Check sheet for the modelled part. Datum: model origin and axes. Units: mm. Face numbers are marked on the shaded views. A direction names the side the tool comes from. Round coordinates to 2 decimals unless told otherwise and drop trailing zeros. Loops run counter-clockwise (first coordinate to the right, second up) from the corner with the lowest first, then second, coordinate; pieces in that order, holes last. Notation, with made-up numbers: (89, 18) - (138, 18) arc R9 ccw to (138, 32) - close; hole circle Ø10 at (-18.5, 52.25). An arc over 180 degrees is marked (long way). Answer in a Markdown table with one row per item. Add a question column.
(1) Mould release check, pull along X, two halves, no side actions. Record for the marked faces 4, 5 and 6: +X half, -X half, draft (parallel to the pull), parting line (faces both ways), or undercut.
(2) Cross-section at B-B on z = 1.35. Enter the section's corners in (x, y).
(3) Thickness scan on line 1 along Y through (x, z) = (-3, 2.1); line 2 along X through (y, z) = (-0.25, 3.3); line 3 along X through (y, z) = (1.75, 1.65). Record the ranges inside material, lowest first.
(4) Cross-section at C-C on y = 9. Enter the section's corners in (x, z), then the cut area to 3 significant figures.
(5) Access from +Z, -Z, +X, -X, +Y, -Y to the whole of each face (thin tool, end or side, straight path). Record for the marked faces 1, 2 and 3.
(6) Cross-section at A-A on x = -1.5. Enter the section's corners in (y, z).
(7) Cross-section at D-D on x = -11.25. Enter the section's corners in (y, z).
(8) Gauge pin test, flat ends, axial feed: pin 1 (9.5 mm diameter, centred on x = 0, y = 0, fed in from -Z); pin 2 (3 mm diameter, centred on x = -4, y = 10, fed in from -Z); pin 3 (1 mm diameter, centred on y = 7.5, z = 2, fed in from +X). Record the tip position at first contact, or that the pin passes through.
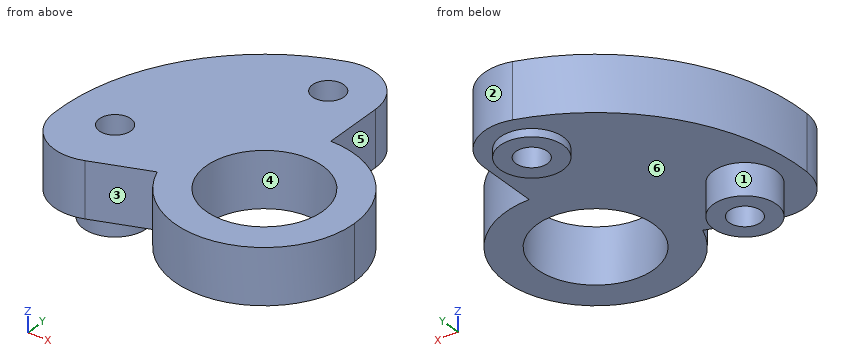
from build123d import *

# Parameters (mm, degrees)
SKETCH1_R           = 13
SKETCH1_R_2         = 5.7
SKETCH1_R_3         = 3.7
BOSS_EXTRUDE1_DEPTH = 3.5
CUT_EXTRUDE1_DEPTH  = 10
SKETCH3_R           = 1
CUT_EXTRUDE2_DEPTH  = 10
SKETCH5_R           = 1
CUT_EXTRUDE3_DEPTH  = 6
FILLET1_R           = 3
SKETCH6_R           = 2
SKETCH6_R_2         = 1
BOSS_EXTRUDE2_DEPTH = 2
SKETCH6_3_R         = 2
SKETCH6_3_R_2       = 1
BOSS_EXTRUDE3_DEPTH = 0.5


with BuildPart() as part:
    # Sketch1 → Boss-Extrude1 (new body)
    with BuildSketch(Plane.XY):
        Circle(SKETCH1_R)
        Circle(SKETCH1_R_2, mode=Mode.SUBTRACT)
        Circle(SKETCH1_R_2)
        Circle(SKETCH1_R_3, mode=Mode.SUBTRACT)
    extrude(amount=BOSS_EXTRUDE1_DEPTH)

    # Sketch2 → Cut-Extrude1 (cut)
    with BuildSketch(Plane.XY.offset(3.5)):
        with BuildLine():
            ThreePointArc((5.7, 0), (0.989794613, -5.613404192), (-5.356247938, -1.949514817))
            Line((-5.356247938, -1.949514817), (-12.21600407, -4.446261863))
            ThreePointArc((-12.21600407, -4.446261863), (2.25742631, -12.802500789), (13, 0))
            ThreePointArc((13, 0), (9.192388155, 9.192388155), (0, 13))
            Line((0, 13), (0, 5.7))
            ThreePointArc((0, 5.7), (4.030508653, 4.030508653), (5.7, 0))
        make_face()
    extrude(amount=-CUT_EXTRUDE1_DEPTH, mode=Mode.SUBTRACT)

    # Sketch3 → Cut-Extrude2 (cut)
    with BuildSketch(Plane.XY.offset(3.5)):
        with Locations((-3, 9.539392014)):
            Circle(SKETCH3_R)
    extrude(amount=-CUT_EXTRUDE2_DEPTH, mode=Mode.SUBTRACT)

    # Sketch5 → Cut-Extrude3 (cut)
    with BuildSketch(Plane.XY.offset(3.5)):
        with Locations((-9.790353578, 0.434714634)):
            Circle(SKETCH5_R)
    extrude(amount=-CUT_EXTRUDE3_DEPTH, mode=Mode.SUBTRACT)

    # Fillet1
    fillet1_edges = [part.edges().sort_by_distance(p)[0] for p in [
        (0, 13, 1.75),
        (-12.21600407, -4.446261863, 1.75),
    ]]
    fillet(fillet1_edges, radius=FILLET1_R)

    # Sketch6 → Boss-Extrude2 (add)
    with BuildSketch(Plane(origin=(0, 0, 0), x_dir=(-1, 0, 0), z_dir=(0, 0, -1))):
        with Locations(Location((9.790353578, 0.434714634, 0), (0, 0, 180))):
            Circle(SKETCH6_R)
        with Locations(Location((9.790353578, 0.434714634, 0), (0, 0, 180))):
            Circle(SKETCH6_R_2, mode=Mode.SUBTRACT)
    extrude(amount=BOSS_EXTRUDE2_DEPTH)

    # Sketch6_3 → Boss-Extrude3 (add)
    with BuildSketch(Plane(origin=(0, 0, 0), x_dir=(-1, 0, 0), z_dir=(0, 0, -1))):
        with Locations(Location((3, 9.539392014, 0), (0, 0, 180))):
            Circle(SKETCH6_3_R)
        with Locations(Location((3, 9.539392014, 0), (0, 0, 180))):
            Circle(SKETCH6_3_R_2, mode=Mode.SUBTRACT)
    extrude(amount=BOSS_EXTRUDE3_DEPTH)


solid = part.part
Answers:
| question | item | result |
|---|---|---|
| 1 | face 4 | undercut |
| 1 | face 5 | +X half |
| 1 | face 6 | draft |
| 2 | outline | (-12.99, -0.58) arc R3 ccw to (-8.96, -3.26) - (-5.36, -1.95) arc R5.7 ccw (long way) to (0, 5.7) - (0, 9.54) arc R3 ccw to (-3.9, 12.4) arc R13 ccw to start; hole circle Ø2 at (-9.79, 0.43); hole circle Ø2 at (-3, 9.54); hole circle Ø7.4 at (0, 0) |
| 3 | line 1 | y = -4.85 to -2.17, 2.17 to 8.54, 10.54 to 12.54 |
| 3 | line 2 | x = -13 to -10.52, -9.06 to -3.69, 3.69 to 5.69 |
| 3 | line 3 | x = -12.88 to -3.26, 3.26 to 5.42 |
| 4 | outline | (-9.38, 0) - (-4.93, 0) - (-4.93, -0.5) - (-3.84, -0.5) - (-3.84, 3.5) - (-9.38, 3.5) - close; (-2.16, -0.5) - (-1.07, -0.5) - (-1.07, 0) - (0, 0) - (0, 3.5) - (-2.16, 3.5) - close |
| 4 | area | 28.0 mm^2 |
| 5 | face 1 | -Z |
| 5 | face 2 | +Z, -Z, +Y |
| 5 | face 3 | +Z, -Z, -Y |
| 6 | outline | (-5.5, 0) - (-3.38, 0) - (-3.38, 3.5) - (-5.5, 3.5) - close; (3.38, 0) - (8.22, 0) - (8.22, -0.5) - (10.86, -0.5) - (10.86, 0) - (12.14, 0) - (12.14, 3.5) - (3.38, 3.5) - close |
| 7 | outline | (-3.17, 0) - (-0.93, 0) - (-0.93, -2) - (1.8, -2) - (1.8, 0) - (6.51, 0) - (6.51, 3.5) - (-3.17, 3.5) - close |
| 8 | pin 1 | stops at z = 0 |
| 8 | pin 2 | stops at z = -0.5 |
| 8 | pin 3 | stops at x = 0 |
